Check sheet for the modelled part. Datum: model origin and axes. Units: mm. Coordinates: 2 decimals unless noted, no trailing zeros. Write each loop counter-clockwise with the first axis right and the second up, starting at its lowest first coordinate (ties: lowest second). Pieces come first, ordered by that corner, then holes. Notation, with made-up numbers: (73.5, 43.25) -> (102.5, 43.25) arc R21 cw to (102.5, 61.25) -> close; hole circle Ø7 at (44, -3). An arc over 180 degrees is marked (long way). One line per item, written item: value. Start each with the question number.
1) Sectioned sample at A-A on z = -155. Enter the section's corners in (x, y), plus the area to 3 significant figures.
2) Scan lines: line 1 along X through (y, z) = (-0.35, 196); line 2 along X through (y, z) = (-0.3, 0); line 3 along Y through (x, z) = (29, 120.5). Record each from-to range of solid material in increasing order. Write a range as [from, to].
3) Gauge pin test, flat end, axial feed: P1, Ø6, axis at x = 7, z = -57, coming from the -Y side. Record the tip position at first contact, or that the pin passes through.
4) Sectioned sample at B-B on x = 14. Enter the section's corners in (y, z), plus the area to 3 significant figures.
```python
from build123d import *

# Parameters (mm, degrees)
SKETCH1_W                    = 37
SKETCH1_H                    = 0.5
BASE_FLANGE1_DEPTH           = 211
SKETCH6_R                    = 1.75
CUT_EXTRUDE1_DEPTH           = 10
EDGE_FLANGE1_STRIP_CUT_DEPTH = 422
EDGE_FLANGE1_DEPTH           = 422
HEM1_START                   = -211
HEM1_DEPTH                   = 422
HEM1_2_DEPTH                 = 422


with BuildPart() as part:
    # Base-Flange1: sheet metal written as solids
    # Sketch1 → Base-Flange1 (new, symmetric)
    with BuildSketch(Plane.XY):
        with Locations((18.5, -0.25)):
            Rectangle(SKETCH1_W, SKETCH1_H)
    extrude(amount=BASE_FLANGE1_DEPTH, both=True)

    # Sketch6 → Cut-Extrude1 (cut)
    with BuildSketch(Plane(origin=(0, 0, 0), x_dir=(1, 0, 0), z_dir=(0, 1, 0))):
        with Locations(Location((5, 196, 0), (0, 0, 270))):
            Circle(SKETCH6_R)
        with Locations(Location((5, 0, 0), (0, 0, 270))):
            Circle(SKETCH6_R)
        with Locations(Location((5, -196, 0), (0, 0, 270))):
            Circle(SKETCH6_R)
    extrude(amount=-CUT_EXTRUDE1_DEPTH, mode=Mode.SUBTRACT)

    # Edge-Flange1: sheet metal written as solids
    # Edge-Flange1 strip (on a plane across the edge) → Edge-Flange1 strip cut (cut)
    with BuildSketch(Plane(origin=(37, -0.5, -211), x_dir=(-0.6560590289905086, 0.754709580222771, 0), z_dir=(0, 0, 1))):
        Polygon((-4.886773951, -6.383716909), (2.13206437, 1.69053295), (1.75470958, 2.018562465), (-5.264128741, -6.055687395), align=None)
    extrude(amount=EDGE_FLANGE1_STRIP_CUT_DEPTH, mode=Mode.SUBTRACT)

    # Edge-Flange1 section (on a plane across the edge) → Edge-Flange1 (add)
    with BuildSketch(Plane(origin=(37, -0.5, -211), x_dir=(-0.6560590289905086, 0.754709580222771, 0), z_dir=(0, 0, 1))):
        with BuildLine():
            Line((-0.5, 2.674621494), (-0.5, 18))
            Line((-0.5, 18), (0, 18))
            Line((0, 18), (0, 2.674621494))
            ThreePointArc((0, 2.674621494), (0.649792619, 1.737949305), (1.75470958, 2.018562465))
            Line((1.75470958, 2.018562465), (2.13206437, 1.69053295))
            ThreePointArc((2.13206437, 1.69053295), (0.474688928, 1.26961321), (-0.5, 2.674621494))
        make_face()
    extrude(amount=EDGE_FLANGE1_DEPTH)

    # Hem1: read off the stored shape, not the designer's step
    # Hem1 outline → Hem1 (cut)
    with BuildSketch(Plane.XY.offset(HEM1_START)):
        with BuildLine():
            ThreePointArc((24.309289256, -12.19437304), (23.892198615, -12.374586092), (23.447599479, -12.280922038))
            Line((23.447599479, -12.280922038), (23.415227556, -12.309062522))
            Line((23.415227556, -12.309062522), (23.74325707, -12.686417312))
            Line((23.74325707, -12.686417312), (24.309289256, -12.19437304))
        make_face()
    extrude(amount=HEM1_DEPTH, mode=Mode.SUBTRACT)

    # Hem1 2 outline → Hem1 2 (add)
    with BuildSketch(Plane.XY.offset(HEM1_START)):
        with BuildLine():
            Line((30.634293844, -5.371117442), (30.306264329, -4.993762652))
            Line((30.306264329, -4.993762652), (23.325200712, -11.06230867))
            ThreePointArc((23.325200712, -11.06230867), (23.070999747, -11.703294486), (23.447599479, -12.280922038))
            Line((23.447599479, -12.280922038), (23.981259741, -11.81701825))
            ThreePointArc((23.981259741, -11.81701825), (23.628567589, -11.792355612), (23.653230227, -11.43966346))
            Line((23.653230227, -11.43966346), (30.634293844, -5.371117442))
        make_face()
    extrude(amount=HEM1_2_DEPTH)


solid = part.part
```
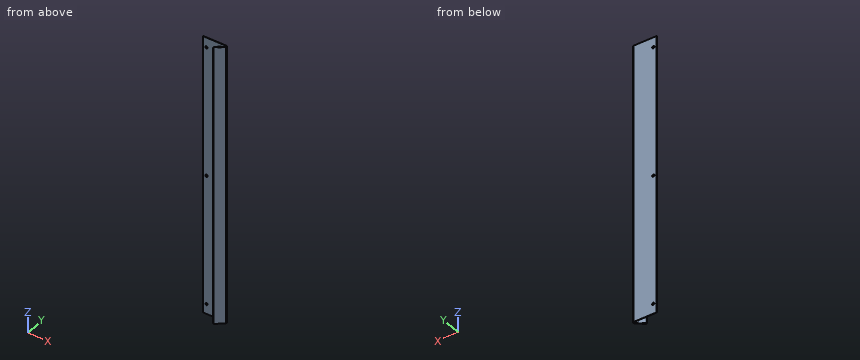
Answers:
1. outline: (0, -0.5) -> (34.33, -0.5) arc R1 cw to (34.98, -2.25) -> (23.98, -11.82) arc R0.25 cw to (23.65, -11.44) -> (30.63, -5.37) -> (30.31, -4.99) -> (23.33, -11.06) arc R0.75 ccw to (24.31, -12.19) -> (35.31, -2.63) arc R1.5 ccw to (34.33, 0) -> (0, 0) -> close
1. area: 31.4 mm2
2. line 1: x = [0, 3.25], [6.75, 35.29]
2. line 2: x = [0, 3.25], [6.75, 35.23]
2. line 3: y = [-8.12, -7.45], [-6.79, -6.13], [-0.5, 0]
3. P1: stops at y = -0.5
4. outline: (-0.5, -211) -> (0, -211) -> (0, 211) -> (-0.5, 211) -> close
4. area: 211 mm2
